Here's how the part is built. I have some questions about the finished solid (model axes, mm). A direction names the side the tool comes from. Coordinates: 2 decimals unless noted, no trailing zeros. Write each loop counter-clockwise with the first axis right and the second up, starting at its lowest first coordinate (ties: lowest second). Pieces come first, ordered by that corner, then holes. Notation, with made-up numbers: (-13, 40.25) -> (20, 40.25) arc R26 cw to (20, 71.25) -> close; hole circle Ø9 at (8.25, -21). An arc over 180 degrees is marked (long way). Put each result on its own line as item: value. Start each with the question number.
Item 1: I want a section at B-B, the plane y = 7.75. List the corners of the cut face in (x, z) for me.
Item 2: I want a section at C-C, the plane z = 7. List the corners of the cut face in (x, y) for me.
Item 3: On a 3-axis mill with a long thin cutter (end or side, diameter ignored), from which of +Z, -Z, +X, -X, +Y, -Y can I reach the whole of each face in a straight line? I mean faces 4 (the face through (29.9, 0, 17.3)), 5 (the face through (0, 13, 49)). Say none if no direction works.
Item 4: For pin 1 (4 mm diameter, centred on x = 38.5, y = 18, fed in from -Z); pin 2 (8 mm diameter, centred on x = 33.5, z = 67.5, fed in from -Y); pin 3 (17 mm diameter, centred on x = 17, z = 9.5, fed in from +Y), each with a flat end and sliding along its axis, tell me the tip position at first contact or that it passes through.
Item 5: I want a section at D-D, the plane z = 58. List the corners of the cut face in (x, y) for me, then the cut area to 3 significant figures.
Item 6: I need wall thicknesses on line 1 (Z direction, x = 3.5, y = 9.25); line 2 (X direction, y = 10.25, z = 12.5); line 3 (Y direction, x = 44.5, z = 78). Which ranges of each line are inside material? Lowest first, please. Write a range as [from, to].
Item 7: If we mould it in two halves opening along Z, with no side actions, what happens to faces 1 (the face through (30, 7, 0)), 2 (the face through (30, 6, 19)), 3 (the face through (30, 13, 9))? For each: released by +Z, released by -Z, zero draft, split by the parting line, or undercut.
from build123d import *

# Parameters (mm, degrees)
BOSS_EXTRUDE1_DEPTH = 17
SKETCH2_W           = 60
SKETCH2_H           = 11
BOSS_EXTRUDE2_DEPTH = 1
BOSS_EXTRUDE3_DEPTH = 64
CUT_EXTRUDE1_DEPTH  = 60
FILLET1_R           = 1


with BuildPart() as part:
    # Sketch1 → Boss-Extrude1 (new body)
    with BuildSketch(Plane.XY):
        Polygon((0, 0), (0, 11), (60, 11), (60, 0), (62, 0), (62, 13), (-2, 13), (-2, 0), align=None)
    extrude(amount=BOSS_EXTRUDE1_DEPTH)

    # Sketch2 → Boss-Extrude2 (add)
    with BuildSketch(Plane(origin=(0, 0, 0), x_dir=(-1, 0, 0), z_dir=(0, 0, -1))):
        with Locations((-30, 5.5)):
            Rectangle(SKETCH2_W, SKETCH2_H)
    extrude(amount=-BOSS_EXTRUDE2_DEPTH)

    # Sketch4 → Boss-Extrude3 (add)
    with BuildSketch(Plane.ZY.offset(2)):
        Polygon((17, 13), (31, 28), (81, 28), (81, 0), (17, 0), align=None)
    extrude(amount=-BOSS_EXTRUDE3_DEPTH)

    # Sketch6 → Cut-Extrude1 (cut)
    with BuildSketch(Plane.ZY):
        Polygon((19, 0), (19, 12.211673639), (31.869104604, 26), (79, 26), (79, 0), align=None)
    extrude(amount=-CUT_EXTRUDE1_DEPTH, mode=Mode.SUBTRACT)

    # Fillet1
    fillet1_edges = [part.edges().sort_by_distance(p)[0] for p in [
        (-2, 0, 40.5),
        (-2, 13, 8.5),
        (62, 13, 8.5),
        (62, 0, 40.5),
        (30, 11, 1),
        (30, 13, 17),
        (62, 20.5, 24),
        (62, 28, 56),
        (30, 28, 31),
        (62, 14, 81),
        (30, 28, 81),
        (30, 0, 81),
        (-2, 14, 81),
        (-2, 28, 56),
        (-2, 20.5, 24),
        (-2, 6.5, 0),
        (30, 13, 0),
        (62, 6.5, 0),
        (30, 0, 0),
    ]]
    fillet(fillet1_edges, radius=FILLET1_R - 0.0001)  # a hair under: the kernel refuses the full size


solid = part.part
Calculated:
1. outline: (-2, 1) arc R1 ccw to (-1, 0) -> (61, 0) arc R1 ccw to (62, 1) -> (62, 80) arc R1 ccw to (61, 81) -> (-1, 81) arc R1 ccw to (-2, 80) -> close; hole (0, 1) -> (60, 1) -> (60, 17) -> (0, 17) -> close; hole (0, 19) -> (60, 19) -> (60, 79) -> (0, 79) -> close
2. outline: (-2, 1) arc R1 ccw to (-1, 0) -> (0, 0) -> (0, 11) -> (60, 11) -> (60, 0) -> (61, 0) arc R1 ccw to (62, 1) -> (62, 12) arc R1 ccw to (61, 13) -> (-1, 13) arc R1 ccw to (-2, 12) -> close
3. face 4: +Z, -Z, +X, -X, -Y
3. face 5: -Y
4. pin 1: stops at z = 19.8
4. pin 2: stops at y = 26
4. pin 3: stops at y = 14.07
5. outline: (-2, 1) arc R1 ccw to (-1, 0) -> (0, 0) -> (0, 26) -> (60, 26) -> (60, 0) -> (61, 0) arc R1 ccw to (62, 1) -> (62, 27) arc R1 ccw to (61, 28) -> (-1, 28) arc R1 ccw to (-2, 27) -> close
5. area: 231 mm2
6. line 1: z = [0, 1], [17, 19], [79, 81]
6. line 2: x = [-2, 0], [60, 62]
6. line 3: y = [26, 28]
7. face 1: released by -Z
7. face 2: undercut
7. face 3: zero draft
